Verification items for this drawing (mm, ordinates from the low corner). Round coordinates to 2 decimals unless told otherwise and drop trailing zeros. Order: outer loops, then holes, each group sorted by start corner. A loop starts at its lowest first (then second) coordinate and runs counter-clockwise, first axis right, second up. Notation, with made-up numbers: (48, 32) -> (59, 32) arc R35 cw to (59, 66) -> close; hole circle Ø11 at (7.25, -16). An arc over 180 degrees is marked (long way). Answer in a Markdown table with one row per item.
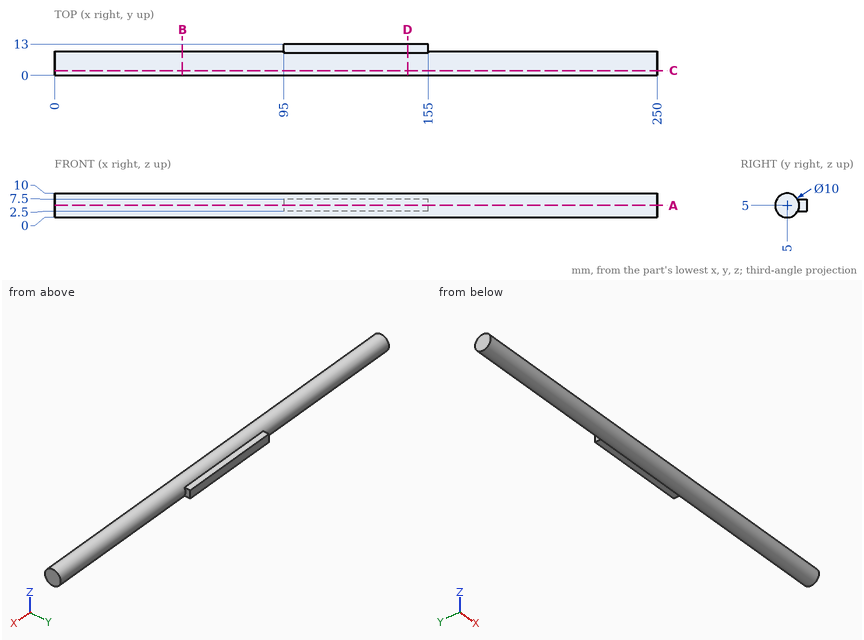
Item 1: Cross-section at B-B (x = 53). Record the boundary of the cut face in (y, z), and give its area (3 significant figures).
Result sheet:
| item | result |
|---|---|
| outline | circle Ø10 at (5, 5) |
| area | 78.5 mm^2 |
Item 2: Cross-section at A-A (z = 5). Record the boundary of the cut face in (x, y).
Result sheet:
| item | result |
|---|---|
| outline | (0, 0) -> (250, 0) -> (250, 10) -> (155, 10) -> (155, 13) -> (95, 13) -> (95, 10) -> (0, 10) -> close |
Item 3: Cross-section at C-C (y = 2). Record the boundary of the cut face in (x, z).
Result sheet:
| item | result |
|---|---|
| outline | (0, 1) -> (250, 1) -> (250, 9) -> (0, 9) -> close |
Item 4: Depth check by flat-ended pin: P1, Ø1.5, axis at y = 11.5, z = 7, coming from the -X side; P2, Ø1.5, axis at x = 202, z = 3, coming from the +Y side; P3, Ø3, axis at x = 179.5, z = 6.5, coming from the -Y side; P4, Ø1.8, axis at y = 11, z = 4.5, coming from the +X side. Enter the tip coordinate at first touch or a pass-through.
Result sheet:
| item | result |
|---|---|
| P1 | stops at x = 95 |
| P2 | stops at y = 9.84 |
| P3 | stops at y = 0 |
| P4 | stops at x = 155 |
Item 5: Cross-section at D-D (x = 146.5). Record the boundary of the cut face in (y, z).
Result sheet:
| item | result |
|---|---|
| outline | (9.33, 2.5) -> (13, 2.5) -> (13, 7.5) -> (9.33, 7.5) arc R5 ccw (long way) to start |
Item 6: Scan lines: line 1 (Z direction, x = 213, y = 4.75); line 2 (X direction, y = 10.75, z = 2.75); line 3 (Y direction, x = 67.5, z = 4). Record each from-to range of solid material in increasing order. Write a range as [from, to].
Result sheet:
| item | result |
|---|---|
| line 1 | z = [0.01, 9.99] |
| line 2 | x = [95, 155] |
| line 3 | y = [0.1, 9.9] |
